Input: part model. Units: mm. Frame: model coordinates. Round coordinates to 2 decimals unless told otherwise and drop trailing zeros. Loops run counter-clockwise (first coordinate to the right, second up) from the corner with the lowest first, then second, coordinate; pieces in that order, holes last. Notation, with made-up numbers: (-18, 84) -> (6, 84) arc R21 ccw to (6, 98) -> close; hole circle Ø11 at (42, 33). An arc over 180 degrees is marked (long way). One line per question, with ' | ' between items. Start each with the question number.
Q1. Contact query for flat-ended pins moving along their axis: P1, Ø1, axis at y = 25, z = 0.5, coming from the -X side; P2, Ø0.6, axis at y = 18.5, z = 1.5, coming from the +X side; P3, Ø1, axis at x = -28, z = 1, coming from the -Y side. Output: stop coordinate, or through.
Q2. Cut plane A-A on z = 1.4. Return loops of the section in (x, y), and give its area (3 significant figures).
Q3. Material intervals for L1, parallel to X at y = 20, z = 1.25; L2, parallel to X at y = 50.5, z = 0.75; L3, parallel to Y at x = 20, z = 1.25, sorted ascending.
Q4. Cut plane C-C on y = 59. Return loops of the section in (x, z), and give its area (3 significant figures).
Q5. Cut plane B-B on x = -7. Return loops of the section in (y, z).
Autodesk Inventor part; units mm, degrees
ref_plane "YZ Plane" through (0, 0, 0) normal (1, 0, 0) x (0, 1, 0)
ref_plane "XZ Plane" through (0, 0, 0) normal (0, 1, 0) x (-1, 0, 0)
ref_plane "XY Plane" through (0, 0, 0) normal (0, 0, 1) x (1, 0, 0)
sketch "Sketch1" plane through (0, 0, 0) normal (0, 0, 1) x (1, 0, 0)
  line L0 (-36, 50) -> (-23.5, 50)
  line L1 (-23.5, 50) -> (-23.5, 0)
  line L2 (-23.5, 0) -> (0, 0)
  arc A0 (0, 86) -> (-36, 50) centre (0, 50) ccw
  line L3 (0, 0) -> (0, 227.422)
  line L4 (0, 50) -> (-63.2946, 50) construction
  line L5 (36, 50) -> (23.5, 50)
  line L6 (23.5, 50) -> (23.5, 0)
  line L7 (23.5, 0) -> (0, 0)
  arc A1 (36, 50) -> (0, 86) centre (0, 50) ccw
  point P0 (0, 0)
  dimension "d4" = 36
  dimension "d5" = 50
  dimension "d6" = 47
extrude "Micromouse1.2.kicad_pcb_Outline" add sketch "Sketch1" along normal blind 2
sketch "Sketch3" plane through (0, 0, 2) normal (0, 0, 1) x (1, 0, 0)
  line L0 (-23.5, 0) -> (23.5, 0)
  line L1 (23.5, 0) -> (23.5, 50)
  line L2 (23.5, 50) -> (36, 50)
  arc A0 (36, 50) -> (-36, 50) centre (0, 50) ccw
  line L3 (-36, 50) -> (-23.5, 50)
  line L4 (-23.5, 50) -> (-23.5, 0)
  line L5 (-57.2581, 25) -> (65.9372, 25)
  line L6 (0, 50) -> (0, -46.1681)
  line L7 (-22, 33.5) -> (-2, 33.5)
  line L8 (-2, 33.5) -> (-2, 16.5)
  line L9 (-2, 16.5) -> (-22, 16.5)
  line L10 (-22, 16.5) -> (-22, 33.5)
  line L11 (22, 33.5) -> (2, 33.5)
  line L12 (2, 33.5) -> (2, 16.5)
  line L13 (2, 16.5) -> (22, 16.5)
  line L14 (22, 16.5) -> (22, 33.5)
  point P0 (0, 0)
  point P1 (-30, 25)
  point P2 (-2, 25)
  dimension "d7" = 25
  dimension "d8" = 17
  dimension "d9" = 20
  dimension "d10" = 4
extrude "Extrusion3" cut sketch "Sketch3" against normal through all contours L10 L7 L8 L5 | L5 L8 L9 L10 | L12 L11 L14 L5 | L5 L14 L13 L12
sketch "Sketch4" plane through (0, 0, 2) normal (0, 0, 1) x (1, 0, 0)
  line L0 (-22, 16.5) -> (-22, 33.5)
  line L1 (-22, 33.5) -> (-2, 33.5)
  line L2 (-2, 33.5) -> (-2, 16.5)
  line L3 (-2, 16.5) -> (-22, 16.5)
  line L4 (22, 33.5) -> (22, 16.5)
  line L5 (22, 16.5) -> (2, 16.5)
  line L6 (2, 16.5) -> (2, 33.5)
  line L7 (2, 33.5) -> (22, 33.5)
  line L8 (-23.5, 0) -> (23.5, 0)
  line L9 (23.5, 0) -> (23.5, 50)
  line L10 (23.5, 50) -> (36, 50)
  arc A0 (36, 50) -> (-36, 50) centre (0, 50) ccw
  line L11 (-36, 50) -> (-23.5, 50)
  line L12 (-23.5, 50) -> (-23.5, 0)
  circle A1 centre (-26, 40) radius 0.5
  line L13 (0, 50) -> (0, -21.7733)
  line L14 (-26, 40) -> (-26, -11.7525) construction
  line L15 (-22, 16.5) -> (-22, 33.5)
  line L16 (-22, 25) -> (-54.7599, 25)
  circle A2 centre (-26, 10) radius 0.5
  circle A3 centre (26, 40) radius 0.5
  circle A4 centre (26, 10) radius 0.5
  point P0 (0, 0)
  dimension "d13" = 1
  dimension "d14" = 52
  dimension "d17" = 30
extrude "Extrusion4" cut sketch "Sketch4" against normal through all contours A1 | A2 | A3 | A4
hole "Hole1" [suppressed]
hole "Hole2" [suppressed]
hole "Hole3" [suppressed]
hole "Hole4" [suppressed]
properties part number "Micromouse_pcb"
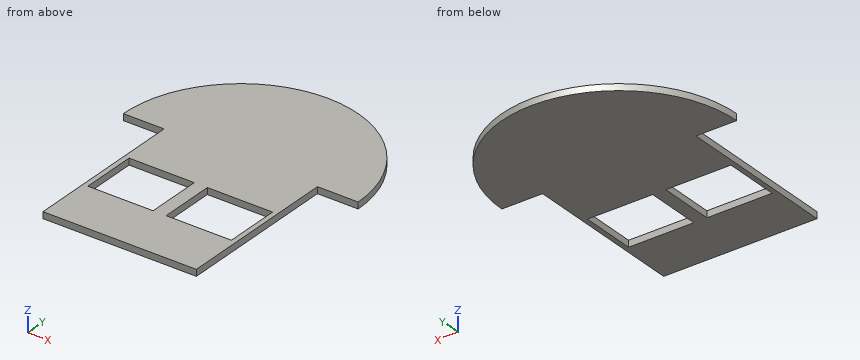
Results:
1) P1: x = -23.5 | P2: x = 23.5 | P3: y = 50
2) outline: (-36, 50) -> (-23.5, 50) -> (-23.5, 0) -> (23.5, 0) -> (23.5, 50) -> (36, 50) arc R36 ccw to start; hole (-22, 16.5) -> (-2, 16.5) -> (-2, 33.5) -> (-22, 33.5) -> close; hole (2, 16.5) -> (22, 16.5) -> (22, 33.5) -> (2, 33.5) -> close | area: 3,710 mm^2
3) L1: -23.5 to -22, -2 to 2, 22 to 23.5 | L2: -36 to 36 | L3: 0 to 16.5, 33.5 to 79.93
4) outline: (-34.86, 0) -> (34.86, 0) -> (34.86, 2) -> (-34.86, 2) -> close | area: 139 mm^2
5) outline: (0, 0) -> (16.5, 0) -> (16.5, 2) -> (0, 2) -> close; (33.5, 0) -> (85.31, 0) -> (85.31, 2) -> (33.5, 2) -> close
